Input: part model. Units: mm. Frame: model coordinates. A direction names the side the tool comes from. Give positions to 0.01 mm unless a question says otherwise; leave off trailing zeros. Order: outer loops, then holes, each group sorted by start corner. A loop starts at its lowest first (then second) coordinate and runs counter-clockwise, first axis right, second up.
```python
from build123d import *

# Parameters (mm, degrees)
BOSS_EXTRUDE1_DEPTH = 10
SKETCH2_R           = 4.5
CUT_EXTRUDE1_DEPTH  = 5
SKETCH3_R           = 3
CUT_EXTRUDE2_DEPTH  = 116.610810509
SKETCH4_R           = 12.5
BOSS_EXTRUDE2_DEPTH = 35
FILLET1_R           = 3


with BuildPart() as part:
    # Sketch1 → Boss-Extrude1 (new body)
    with BuildSketch(Plane(origin=(0, 0, 0), x_dir=(1, 0, 0), z_dir=(0, 1, 0))):
        with BuildLine():
            Line((-10.825317547, -6.25), (-55.807953086, 71.662210211))
            ThreePointArc((-55.807953086, 71.662210211), (-56.841976003, 79.115981661), (-52.386332276, 85.180233568))
            ThreePointArc((-52.386332276, 85.180233568), (0, 100), (52.386332276, 85.180233568))
            ThreePointArc((52.386332276, 85.180233568), (56.841976003, 79.115981661), (55.807953086, 71.662210211))
            Line((55.807953086, 71.662210211), (10.825317547, -6.25))
            ThreePointArc((10.825317547, -6.25), (0, -12.5), (-10.825317547, -6.25))
        make_face()
    extrude(amount=BOSS_EXTRUDE1_DEPTH)

    # Sketch2 → Cut-Extrude1 (cut)
    with BuildSketch(Plane(origin=(0, 10, 0), x_dir=(1, 0, 0), z_dir=(0, 1, 0))):
        with Locations(Location((10, 28.284271247, 0), (0, 0, 270))):
            Circle(SKETCH2_R)
        with Locations(Location((-10, 28.284271247, 0), (0, 0, 90))):
            Circle(SKETCH2_R)
    extrude(amount=-CUT_EXTRUDE1_DEPTH, mode=Mode.SUBTRACT)

    # Sketch3 → Cut-Extrude2 (cut, through all)
    with BuildSketch(Plane(origin=(0, 10, 0), x_dir=(1, 0, 0), z_dir=(0, 1, 0))):
        with Locations(Location((10, 28.284271247, 0), (0, 0, 270))):
            Circle(SKETCH3_R)
        with Locations(Location((-10, 28.284271247, 0), (0, 0, 90))):
            Circle(SKETCH3_R)
    extrude(amount=-CUT_EXTRUDE2_DEPTH, mode=Mode.SUBTRACT)

    # Sketch4 → Boss-Extrude2 (add)
    with BuildSketch(Plane(origin=(0, 10, 0), x_dir=(1, 0, 0), z_dir=(0, 1, 0))):
        with Locations(Location((0, 0, 0), (0, 0, 330))):
            Circle(SKETCH4_R)
    extrude(amount=BOSS_EXTRUDE2_DEPTH)

    # Fillet1
    fillet1_edges = [part.edges().sort_by_distance(p)[0] for p in [
        (-10.825317547, 45, -6.25),
    ]]
    fillet(fillet1_edges, radius=FILLET1_R)


solid = part.part
```
1) Cut plane C-C (y = 20). Return the cut outline in (x, z).
2) Reachability of faces 4 (the face through (0, 45, 0)), 5 (the face through (-13.041, 7.535, -24.968)) from +Z, -Z, +X, -X, +Y, -Y: full face, straight path, thin tool, end or side. Return the list, or none.
3) Pull-direction query (Z, two-part tool) for faces 1 (the face through (-33, 4.93, -32.16)), 2 (the face through (-0.772, 4.93, -99.997)), 3 (the face through (-7, 5, -27)); classes: pulls with the +Z half, pulls with the -Z half, needs draft (parallel to the pull), parting line crosses it, or undercut.
4) Cut plane A-A (y = 8). Return the cut outline in (x, z), then the cut area to 3 significant figures.
5) Cut plane D-D (x = 17.5). Return the cut outline in (y, z), then the cut area to 3 significant figures.
6) Cut plane B-B (z = 0). Return the cut outline in (x, y).
7) First-contact query: P1, Ø4, axis at x = 10.5, y = 39.5, coming from the -Z side; P2, Ø10, axis at x = 13, y = 22.5, coming from the +Z side; P3, Ø4.5, axis at x = 10, z = -29, coming from the +Y side; P4, Ø7, axis at x = -10, z = -28.28, coming from the +Y side. Flat tips, straight axial feed; report the tip coordinate or a pass-through.
8) Line query: probe 1 along Y at (x, z) = (-7, -46); probe 2 along Z at (x, y) = (-10, 3); probe 3 along Z at (x, y) = (41, 3). Output: solid intervals per line, ascending.
Geometry says:
1. outline: circle Ø25 at (0, 0)
2. face 4: +Z, -Z, +X, -X, +Y
2. face 5: +Y
3. face 1: pulls with the +Z half
3. face 2: pulls with the -Z half
3. face 3: undercut
4. outline: (-55.81, -71.66) arc R10 ccw to (-52.39, -85.18) arc R100 ccw to (52.39, -85.18) arc R10 ccw to (55.81, -71.66) - (10.83, 6.25) arc R12.5 ccw to (-10.83, 6.25) - close; hole circle Ø9 at (-10, -28.28); hole circle Ø9 at (10, -28.28)
4. area: 7,730 mm2
5. outline: (0, -98.46) - (10, -98.46) - (10, -5.31) - (0, -5.31) - close
5. area: 931 mm2
6. outline: (-14.43, 0) - (14.43, 0) - (14.43, 10) - (12.5, 10) - (12.5, 42) arc R3 ccw to (9.5, 45) - (-9.5, 45) arc R3 ccw to (-12.5, 42) - (-12.5, 10) - (-14.43, 10) - close
7. P1: stops at z = -9.17
7. P2: stops at z = 9.6
7. P3: passes through
7. P4: stops at y = 5
8. probe 1: y = 0 to 10
8. probe 2: z = -99.5 to -31.28, -25.28 to 7.5
8. probe 3: z = -91.21 to -46.01
